from build123d import *

# Parameters (mm, degrees)
SKETCH_R     = 3.8
PAD_DEPTH    = 18
SKETCH001_R  = 2.25
POCKET_DEPTH = 14.5
FILLET_R     = 2


with BuildPart() as part:
    # Sketch → Pad (new body)
    with BuildSketch(Plane.XY):
        Circle(SKETCH_R)
    extrude(amount=PAD_DEPTH)

    # Sketch001 (on Face3 of Pad) → Pocket (cut)
    with BuildSketch(Plane.XY.offset(18)):
        Circle(SKETCH001_R)
    extrude(amount=-POCKET_DEPTH, mode=Mode.SUBTRACT)

    # Fillet
    fillet_edges = [part.edges().sort_by_distance(p)[0] for p in [
        (-3.8, 0, 0),
    ]]
    fillet(fillet_edges, radius=FILLET_R)


solid = part.part
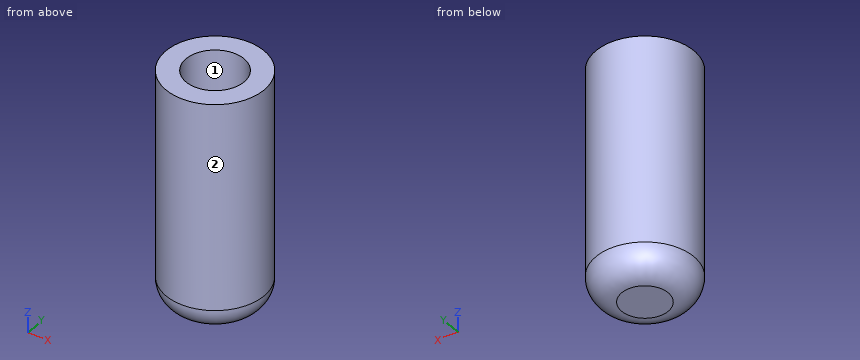
Here's how the part is built. I have some questions about the finished solid (model axes, mm). Face numbers are marked on the shaded views. A direction names the side the tool comes from. Give positions to 0.01 mm unless a question says otherwise; leave off trailing zeros. Loops run counter-clockwise (first coordinate to the right, second up) from the corner with the lowest first, then second, coordinate; pieces in that order, holes last. Notation, with made-up numbers: (5.25, 58.25) -> (41.25, 58.25) arc R13 ccw to (41.25, 81.25) -> close; hole circle Ø8 at (8, -10.5). An arc over 180 degrees is marked (long way). One line per item, written item: value.
Q1. If I drill on line 1 along Y through (x, z) = (0, 12.5); line 2 along Z through (x, y) = (-1.5, -0.25); line 3 along Y through (x, z) = (-1.25, 10), over which ranges is the centre line in solid material (lowest first)?
Answers follow:
line 1: -3.8 to -2.25, 2.25 to 3.8
line 2: 0 to 3.5
line 3: -3.59 to -1.87, 1.87 to 3.59
Q2. Suppose I cut it at A-A on z = 12. Please give me the cut outline in (x, y).
Answers follow:
outline: circle Ø7.6 at (0, 0); hole circle Ø4.5 at (0, 0)
Q3. On a 3-axis mill with a long thin cutter (end or side, diameter ignored), from which of +Z, -Z, +X, -X, +Y, -Y can I reach the whole of each face in a straight line? I mean the marked faces 1 and 2. Say none if no direction works.
Answers follow:
face 1: +Z
face 2: +Z, -Z
Q4. I'm going to push flat-ended pins straight in: pin 1 Ø4 at (x, z) = (2.5, 8.5) entering from -Y; pin 2 Ø1 at (x, z) = (-1.5, 13) entering from +Y; pin 3 Ø2.5 at (x, y) = (0, 0) entering from +Z. Where does each tip first touch, or does it pass through?
Answers follow:
pin 1: y = -3.77
pin 2: y = 3.67
pin 3: z = 3.5
